```python
from build123d import *

# Parameters (mm, degrees)
DODANIE_WYCI_GNI_CIE1_DEPTH = 4
DODANIE_WYCI_GNI_CIE2_DEPTH = 0.5
WYTNIJ_WYCI_GNI_CIE6_DEPTH  = 4
WYTNIJ_WYCI_GNI_CIE7_DEPTH  = 10
SZKIC8_R                    = 1.75
WYTNIJ_WYCI_GNI_CIE8_DEPTH  = 10
SZKIC9_R                    = 0.75
WYTNIJ_WYCI_GNI_CIE9_DEPTH  = 10


with BuildPart() as part:
    # Szkic1 → Dodanie-wyciągnięcie1 (new body)
    with BuildSketch(Plane(origin=(0, 0, 0), x_dir=(1, 0, 0), z_dir=(0, 1, 0))):
        with BuildLine():
            Line((-7.225110555, 24.972122297), (-9.998428156, 2.972122297))
            ThreePointArc((-9.998428156, 2.972122297), (0, -10.430823387), (9.998428156, 2.972122297))
            Line((9.998428156, 2.972122297), (7.225110555, 24.972122297))
            ThreePointArc((7.225110555, 24.972122297), (0, 32.183793132), (-7.225110555, 24.972122297))
        make_face()
        with BuildLine():
            Line((-5.067752367, 2.972122297), (-3.003681195, 14.820995555))
            Line((-3.003681195, 14.820995555), (-2.892810316, 16.996498506))
            ThreePointArc((-2.892810316, 16.996498506), (0, 19.989966002), (2.892810316, 16.996498506))
            Line((2.892810316, 16.996498506), (2.962451003, 14.820995555))
            Line((2.962451003, 14.820995555), (5.067752367, 2.972122297))
            ThreePointArc((5.067752367, 2.972122297), (0, -5.875), (-5.067752367, 2.972122297))
        make_face(mode=Mode.SUBTRACT)
    extrude(amount=DODANIE_WYCI_GNI_CIE1_DEPTH)

    # Szkic2 → Dodanie-wyciągnięcie2 (add)
    with BuildSketch(Plane(origin=(0, 4, 0), x_dir=(1, 0, 0), z_dir=(0, 1, 0))):
        with BuildLine():
            Line((-7.225110555, 24.972122297), (-9.998428156, 2.972122297))
            ThreePointArc((-9.998428156, 2.972122297), (0, -10.430823387), (9.998428156, 2.972122297))
            Line((9.998428156, 2.972122297), (7.225110555, 24.972122297))
            ThreePointArc((7.225110555, 24.972122297), (0, 32.183793132), (-7.225110555, 24.972122297))
        make_face()
    extrude(amount=DODANIE_WYCI_GNI_CIE2_DEPTH)

    # Szkic5 → Wytnij-wyciągnięcie6 (cut)
    with BuildSketch(Plane.XZ):
        with BuildLine():
            Line((-2.212371502, 17.095463356), (2.237628498, 17.095463356))
            Line((2.237628498, 17.095463356), (4.534426812, 3.735585428))
            ThreePointArc((4.534426812, 3.735585428), (0.000881881, 5.874999934), (-4.53330513, 3.736946561))
            Line((-4.53330513, 3.736946561), (-2.212371502, 17.095463356))
        make_face()
    extrude(amount=-WYTNIJ_WYCI_GNI_CIE6_DEPTH, mode=Mode.SUBTRACT)

    # Szkic7 → Wytnij-wyciągnięcie7 (cut)
    with BuildSketch(Plane.XZ):
        with BuildLine():
            Line((-9.294248657, 4.73487259), (9.297326284, 4.728826547))
            ThreePointArc((9.297326284, 4.728826547), (0.003392139, 10.430822836), (-9.294248657, 4.73487259))
        make_face()
    extrude(amount=-WYTNIJ_WYCI_GNI_CIE7_DEPTH, mode=Mode.SUBTRACT)

    # Szkic8 → Wytnij-wyciągnięcie8 (cut)
    with BuildSketch(Plane.XZ):
        with Locations(Location((0, -25.563793132, 0), (0, 0, 270))):
            Circle(SZKIC8_R)
    extrude(amount=-WYTNIJ_WYCI_GNI_CIE8_DEPTH, mode=Mode.SUBTRACT)

    # Szkic9 → Wytnij-wyciągnięcie9 (cut)
    with BuildSketch(Plane.XZ.offset(-4)):
        with Locations(Location((0, -16.003793132, 0), (0, 0, 270))):
            Circle(SZKIC9_R)
        with Locations(Location((0, -13.003793132, 0), (0, 0, 270))):
            Circle(SZKIC9_R)
        with Locations(Location((0, -10.003793132, 0), (0, 0, 270))):
            Circle(SZKIC9_R)
        with Locations(Location((0, -7.003793132, 0), (0, 0, 270))):
            Circle(SZKIC9_R)
    extrude(amount=-WYTNIJ_WYCI_GNI_CIE9_DEPTH, mode=Mode.SUBTRACT)


solid = part.part
```
Part model, mm, in its own coordinate system. A direction names the side the tool comes from. Coordinates: 2 decimals unless noted, no trailing zeros. Write each loop counter-clockwise with the first axis right and the second up, starting at its lowest first coordinate (ties: lowest second). Pieces come first, ordered by that corner, then holes.
Item 1: Slice it at D-D (x = 8.75). Write the cut outline in (y, z), and give its area (3 significant figures).
Item 2: Slice it at B-B (x = 0). Write the cut outline in (y, z), and give its area (3 significant figures).
Item 3: Probe line 1 (Y direction, x = 0.5, z = -18.5); line 2 (X direction, y = 1.45, z = 0) (3 decimals); line 3 (X direction, y = 1.45, z = -7). List the from-to ranges inside material, lowest first.
Item 4: Pin check, flat tips, straight feed: pin 1 (1.5 mm diameter, centred on x = -6.5, y = 2, fed in from -Z); pin 2 (0.9 mm diameter, centred on x = 0, z = -16, fed in from +Y); pin 3 (1.5 mm diameter, centred on y = 3.5, z = -25.5, fed in from -X); pin 4 (1 mm diameter, centred on x = -7, z = -7.5, fed in from -Y). Stop position of each tip, or through.
Item 5: Which spindle directions (+Z, -Z, +X, -X, +Y, -Y) get a long thin tool onto all of the face, cutting with end or side? Do faces 1 (the face through (-4.05, 1.97, -8.81)), 2 (the face through (0.159, 2.218, -32.182)). Say none if no direction does.
Item 6: Mould opens along Z. For faces 3 (the face through (-4.448, 1.972, 4.228)), 4 (the face through (-10.392, 2.218, 0.894)), 5 (the face through (-2.95, 1.97, -15.89)) say: released by +Z, released by -Z, zero draft, split by the parting line, or undercut.
Item 7: Slice it at C-C (z = -26.5). Write the cut outline in (x, y), and give its area (3 significant figures).
Results found:
1. outline: (0, -12.88) - (4.5, -12.88) - (4.5, 4.73) - (0, 4.73) - close
1. area: 79.2 mm2
2. outline: (0, -32.18) - (4.5, -32.18) - (4.5, -27.31) - (0, -27.31) - close; (0, -23.81) - (4.5, -23.81) - (4.5, -16.75) - (4, -16.75) - (4, -19.99) - (0, -19.99) - close; (4, -15.25) - (4.5, -15.25) - (4.5, -13.75) - (4, -13.75) - close; (4, -12.25) - (4.5, -12.25) - (4.5, -10.75) - (4, -10.75) - close; (4, -9.25) - (4.5, -9.25) - (4.5, -7.75) - (4, -7.75) - close; (4, -6.25) - (4.5, -6.25) - (4.5, 4.73) - (4, 4.73) - close
2. area: 48.5 mm2
3. line 1: y = 4 to 4.5
3. line 2: x = -10.431 to -5.875, 5.875 to 10.431
3. line 3: x = -9.49 to -4.37, 4.35 to 9.49
4. pin 1: stops at z = -29.33
4. pin 2: passes through
4. pin 3: stops at x = -7.25
4. pin 4: stops at y = 0
5. face 1: -Y
5. face 2: -Z, +Y, -Y
6. face 3: undercut
6. face 4: split by the parting line
6. face 5: released by +Z
7. outline: (-7.06, 0) - (-1.48, 0) - (-1.48, 4.5) - (-7.06, 4.5) - close; (1.48, 0) - (7.06, 0) - (7.06, 4.5) - (1.48, 4.5) - close
7. area: 50.2 mm2
